from build123d import *

# Parameters (mm, degrees)
ESQUISSE1_R      = 9
EXTRUSION1_DEPTH = 1.6


with BuildPart() as part:
    # Esquisse1 → Extrusion1 (new body)
    with BuildSketch(Plane(origin=(0, 0, 0), x_dir=(1, 0, 0), z_dir=(0, 1, 0))):
        with BuildLine():
            Line((-24, 9), (-24, -29))
            Line((-24, -29), (18, -29))
            Line((18, -29), (18, -13))
            ThreePointArc((18, -13), (22.416407865, -7.708203932), (24, -1))
            Line((24, -1), (24, 9))
            ThreePointArc((24, 9), (18.793114224, 23.078458513), (5, 29))
            Line((5, 29), (-5, 29))
            ThreePointArc((-5, 29), (-18.793114224, 23.078458513), (-24, 9))
        make_face()
        with Locations(Location((0, 6, 0), (0, 0, 270))):
            Circle(ESQUISSE1_R, mode=Mode.SUBTRACT)
    extrude(amount=EXTRUSION1_DEPTH)


solid = part.part
The listing builds one solid part. Answer for the finished solid, in the listing's coordinates (mm). A direction names the side the tool comes from. Give positions to 0.01 mm unless a question says otherwise; leave off trailing zeros. Order: outer loops, then holes, each group sorted by start corner. A loop starts at its lowest first (then second) coordinate and runs counter-clockwise, first axis right, second up. Notation, with made-up numbers: (-34, 80) - (25, 80) arc R19 ccw to (25, 115) - close; hole circle Ø7 at (12, -14). An arc over 180 degrees is marked (long way). Use one line per item in the form item = value.
1) For faces 4 (the flat face through (18, 1, 21)), 5 (the flat face through (0, 1.6, 6)), determine the directions among +Z, -Z, +X, -X, +Y, -Y from which every point of the face is accessible in a straight line to the end or side of a thin tool.
Verdict:
face_4 = +Z, +X, +Y, -Y
face_5 = +Z, -Z, +X, -X, +Y
2) Find section B-B on y = 0.5. Determine the outline of the cut face in (x, z) (3 decimals), and give its area (3 significant figures).
Verdict:
outline = (-24, -9) arc R19.025 ccw to (-5, -29) - (5, -29) arc R19.025 ccw to (24, -9) - (24, 1) arc R15 ccw to (18, 13) - (18, 29) - (-24, 29) - close; hole circle Ø18 at (0, -6)
area = 2,260 mm^2
3) Find section A-A on x = 0. Determine the outline of the cut face in (y, z).
Verdict:
outline = (0, -29) - (1.6, -29) - (1.6, -15) - (0, -15) - close; (0, 3) - (1.6, 3) - (1.6, 29) - (0, 29) - close
4) The mould has two halves that part along X. Classify faces 1 (the cylindrical face through (18.94, 0.79, -22.92)), 2 (the flat face through (0, 1, -29)), 3 (the cylindrical face through (2.703, 0.789, 2.584)): released by +X, released by -X, zero draft, split by the parting line, or undercut.
Verdict:
face_1 = released by +X
face_2 = zero draft
face_3 = undercut
5) Find section C-C on z = -6. Determine the outline of the cut face in (x, y).
Verdict:
outline = (-24, 0) - (-9, 0) - (-9, 1.6) - (-24, 1.6) - close; (9, 0) - (24, 0) - (24, 1.6) - (9, 1.6) - close
6) Consider probe 1 along X at (y, z) = (1, -6); probe 2 along Z at (x, y) = (-0.5, 1.3); probe 3 along X at (y, z) = (1.15, -4). Determine where each line is inside the solid, lowest interval first. Write a range as [from, to].
Verdict:
probe_1 = [-24, -9], [9, 24]
probe_2 = [-29, -14.99], [2.99, 29]
probe_3 = [-24, -8.77], [8.77, 24]
7) Find section D-D on z = 17. Determine the outline of the cut face in (x, y), and give its area (3 significant figures).
Verdict:
outline = (-24, 0) - (18, 0) - (18, 1.6) - (-24, 1.6) - close
area = 67.2 mm^2
8) Each of these flat-tipped pins is pushed along its axis until it touches: pin 1 (20.5 mm diameter, centred on x = 0, z = -6, fed in from +Y); pin 2 (0.5 mm diameter, centred on y = 1, z = -5, fed in from +X); pin 3 (0.5 mm diameter, centred on y = 1, z = 18, fed in from +X). Where does it stop, or does it pass through?
Verdict:
pin_1 = 1.6
pin_2 = 24
pin_3 = 18
